Answer from the drawing. Dimensions are ordinates in mm from the lowest x, y and z of the part. A direction names the side the tool comes from. Round coordinates to 2 decimals unless told otherwise and drop trailing zeros. Write each loop counter-clockwise with the first axis right and the second up, starting at its lowest first coordinate (ties: lowest second). Pieces come first, ordered by that corner, then holes. Notation, with made-up numbers: (51.25, -31) -> (110.25, -31) arc R21 cw to (110.25, -19) -> close; hole circle Ø9 at (-32.75, 7.25). An arc over 180 degrees is marked (long way). Answer as a JSON object with one key per item and string values. Group by question number.
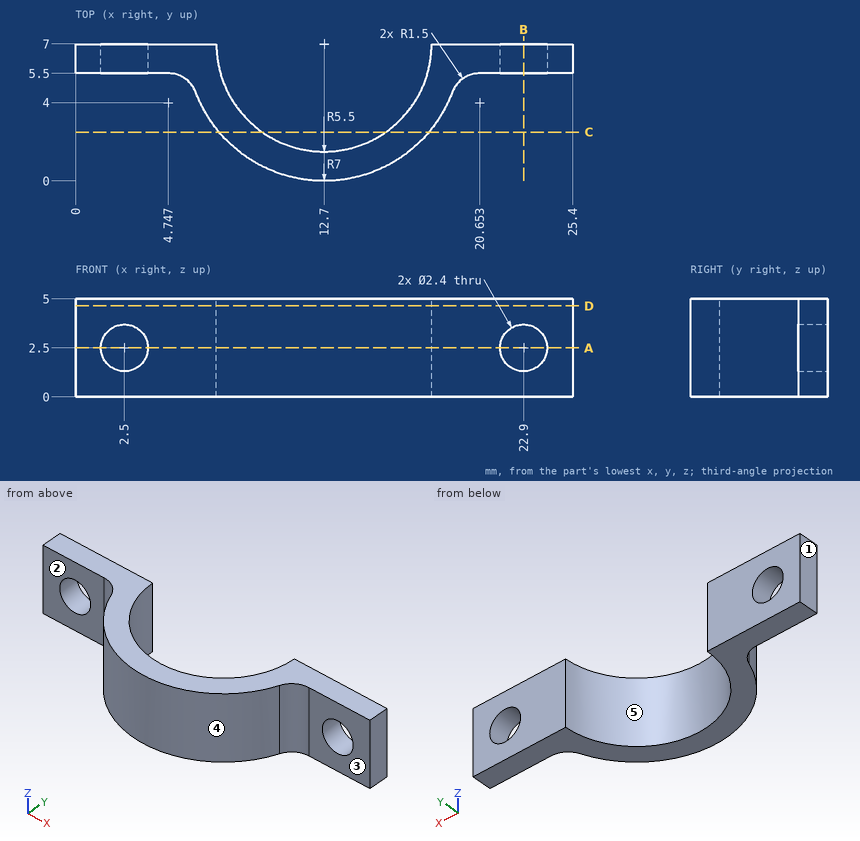
1) Each of these flat-tipped pins is pushed along its axis until it touches: P1, Ø1.5, axis at x = 13.5, z = 1, coming from the +Y side; P2, Ø1, axis at x = 9.5, z = 2.5, coming from the -Y side; P3, Ø1.4, axis at x = 23, z = 1.5, coming from the -Y side. Where does it stop, or does it pass through?
2) For a pull along X with two mould halves and no side action, classify the marked faces 3, 4 and 5 as released by +X, released by -X, zero draft, split by the parting line, or undercut.
3) A cutting plane is placed at A-A on z = 2.5. Determine the outline of the cut face in (x, y).
4) A cutting plane is placed at C-C on y = 2.5. Determine the outline of the cut face in (x, z), plus the area to 3 significant figures.
5) A tool of negligible diameter and unlimited length cuts with its end or side. For the marked faces 1 and 2, from which of +Z, -Z, +X, -X, +Y, -Y can it reach the whole face along a straight path? Write none if from no direction.
6) Straight lines are drawn through the part: L1, parallel to Z at x = 22.9, y = 6.35; L2, parallel to X at y = 6.15, z = 2.5; L3, parallel to Y at x = 1.75, z = 3.95. For each, find the intervals that lie inside material, in ascending order.
7) A cutting plane is placed at D-D on z = 4.65. Determine the outline of the cut face in (x, y).
8) A cutting plane is placed at B-B on x = 22.9. Determine the outline of the cut face in (y, z), plus the area to 3 significant figures.
Established:
{
 "1": {"P1": "stops at y = 1.72", "P2": "stops at y = 0.54", "P3": "stops at y = 5.5"},
 "2": {"face 3": "zero draft", "face 4": "split by the parting line", "face 5": "undercut"},
 "3": {"outline": "(0, 5.5) -> (1.3, 5.5) -> (1.3, 7) -> (0, 7) -> close; (3.7, 5.5) -> (4.75, 5.5) arc R1.5 cw to (6.15, 4.53) arc R7 ccw to (19.25, 4.53) arc R1.5 cw to (20.65, 5.5) -> (21.7, 5.5) -> (21.7, 7) -> (18.2, 7) arc R5.5 cw to (7.2, 7) -> (3.7, 7) -> close; (24.1, 5.5) -> (25.4, 5.5) -> (25.4, 7) -> (24.1, 7) -> close"},
 "4": {"outline": "(7.34, 0) -> (9.54, 0) -> (9.54, 5) -> (7.34, 5) -> close; (15.86, 0) -> (18.06, 0) -> (18.06, 5) -> (15.86, 5) -> close", "area": "22.0 mm²"},
 "5": {"face 1": "+Z, -Z, -X, +Y, -Y", "face 2": "+Z, -Z, -X, -Y"},
 "6": {"L1": "z = 0 to 1.3, 3.7 to 5", "L2": "x = 0 to 1.3, 3.7 to 7.27, 18.13 to 21.7, 24.1 to 25.4", "L3": "y = 5.5 to 7"},
 "7": {"outline": "(0, 5.5) -> (4.75, 5.5) arc R1.5 cw to (6.15, 4.53) arc R7 ccw to (19.25, 4.53) arc R1.5 cw to (20.65, 5.5) -> (25.4, 5.5) -> (25.4, 7) -> (18.2, 7) arc R5.5 cw to (7.2, 7) -> (0, 7) -> close"},
 "8": {"outline": "(5.5, 0) -> (7, 0) -> (7, 1.3) -> (5.5, 1.3) -> close; (5.5, 3.7) -> (7, 3.7) -> (7, 5) -> (5.5, 5) -> close", "area": "3.90 mm²"}
}
